```python
from build123d import *

# Parameters (mm, degrees)
F0_W      = 30
F0_H      = 30
F1_DEPTH  = 600
F2_W      = 460
F2_H      = 270
F3_DEPTH  = 25
F5_DEPTH  = 30
F7_DEPTH  = 30
F9_DEPTH  = 30
F11_DEPTH = 30


with BuildPart() as f1:
    # F0 (on Top) → F1 (new body)
    with BuildSketch(Plane.XY):
        with Locations((-215, 120)):
            Rectangle(F0_W, F0_H)
    extrude(amount=-F1_DEPTH)



with BuildPart() as f1b:
    # F0 (on Top) → F1, piece 2 (new body)
    with BuildSketch(Plane.XY):
        with Locations((-215, -120)):
            Rectangle(F0_W, F0_H)
    extrude(amount=-F1_DEPTH)


with BuildPart() as f1c:
    # F0 (on Top) → F1, piece 3 (new body)
    with BuildSketch(Plane.XY):
        with Locations((215, 120)):
            Rectangle(F0_W, F0_H)
    extrude(amount=-F1_DEPTH)


with BuildPart() as f1d:
    # F0 (on Top) → F1, piece 4 (new body)
    with BuildSketch(Plane.XY):
        with Locations((215, -120)):
            Rectangle(F0_W, F0_H)
    extrude(amount=-F1_DEPTH)


with BuildPart() as f1_1:
    add(f1.part)

    add(f1b.part)  # F3 merges F1b

    add(f1c.part)  # F3 merges F1c

    add(f1d.part)  # F3 merges F1d
    # F2 (on face) → F3 (join)
    with BuildSketch(Plane.XY):
        Rectangle(F2_W, F2_H)
    extrude(amount=-F3_DEPTH)

    # F4 (on face) → F5 (join)
    with BuildSketch(Plane.XZ.offset(135)):
        Polygon((-200, -25), (-200, -66.8888936143), (200, -562.8062018801), (200, -513.5346421648), (-194.0452442551, -25), align=None)
    extrude(amount=-F5_DEPTH)

    # F6 (on face) → F7 (join)
    with BuildSketch(Plane.XZ.offset(-105)):
        Polygon((-214.2098963722, 0), (-230, -29.6950954944), (230, -600), (230, -550.7284402847), align=None)
    extrude(amount=-F7_DEPTH)

    # F8 (on face) → F9 (join)
    with BuildSketch(Plane(origin=(-230, 0, 0), x_dir=(0, -1, 0), z_dir=(-1, 0, 0))):
        Polygon((-105, -25), (-105, -75), (105, -600), (105, -525), (-95, -25), align=None)
    extrude(amount=-F9_DEPTH)

    # F10 (on face) → F11 (join)
    with BuildSketch(Plane.YZ.offset(230)):
        Polygon((95, -25), (-105, -525), (-105, -600), (105, -75), (105, -25), align=None)
    extrude(amount=-F11_DEPTH)


solid = f1_1.part
```
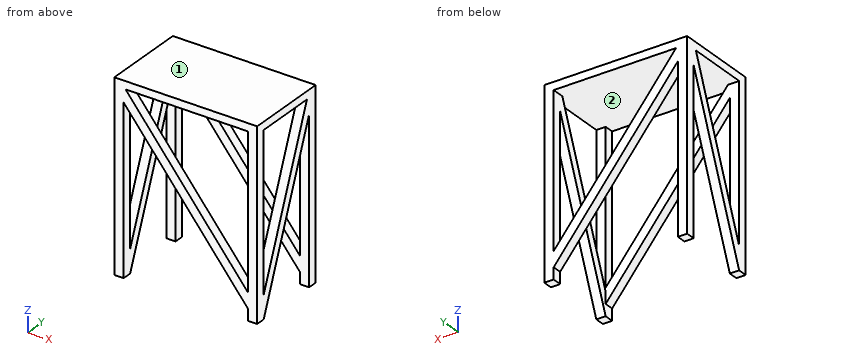
Build history of the part. All positions in model axes, mm. Face numbers are marked on the shaded views. Give positions to 0.01 mm unless a question says otherwise; leave off trailing zeros. Loops run counter-clockwise (first coordinate to the right, second up) from the corner with the lowest first, then second, coordinate; pieces in that order, holes last.
Item 1: Pull direction X, two halves, no side cores. Call the marked faces 1 and 2: released by +X, released by -X, zero draft, split by the parting line, or undercut.
Answers follow:
face 1: zero draft
face 2: undercut
Item 2: Slice it at D-D, the plane z = -409.5. Give the number of separate pieces and of enclosed holes in the cut face, and give its area (3 significant figures).
Answers follow:
separate pieces: 8
enclosed holes: 0
area: 7,780 mm2
Item 3: Slice it at B-B, the plane z = -49. List the corners of the cut face in (x, y).
Answers follow:
outline: (-230, -135) - (-174.69, -135) - (-174.69, -105) - (-230, -105) - close; (-230, 85.4) - (-200, 85.4) - (-200, 105) - (-174.69, 105) - (-174.69, 135) - (-230, 135) - close; (200, -135) - (230, -135) - (230, -105) - (200, -105) - close; (200, 85.4) - (230, 85.4) - (230, 135) - (200, 135) - close
Item 4: Slice it at C-C, the plane x = 98.5. List the corners of the cut face in (y, z).
Answers follow:
outline: (-135, -436.97) - (-105, -436.97) - (-105, -387.7) - (-135, -387.7) - close; (-135, -25) - (135, -25) - (135, 0) - (-135, 0) - close; (105, -436.97) - (135, -436.97) - (135, -387.7) - (105, -387.7) - close
Item 5: Slice it at A-A, the plane y = -91.5. List the corners of the cut face in (x, z).
Answers follow:
outline: (-230, -566.25) - (-200, -566.25) - (-200, -491.25) - (-230, -491.25) - close; (-230, -25) - (230, -25) - (230, 0) - (-230, 0) - close; (200, -566.25) - (230, -566.25) - (230, -491.25) - (200, -491.25) - close
Item 6: Drill centre lines: line 1 (Y direction, x = 66, z = -360.5); line 2 (X direction, y = -21, z = -360.5); line 3 (X direction, y = 116, z = -478.5). Where is each one in solid material? Low to high.
Answers follow:
line 1: y = -135 to -105, 105 to 135
line 2: x = -230 to -200, 200 to 230
line 3: x = -230 to -200, 132 to 171.74, 200 to 230
Item 7: Flat gauge pin, fed straight in: pin 1 (4 mm diameter, centred on x = -141.5, y = 34.5, fed in from -Z). Where does the tip first touch, or does it go through?
Answers follow:
pin 1: stops at z = -25
